Autodesk Inventor part; units mm, degrees
ref_plane "YZ Plane" through (0, 0, 0) normal (1, 0, 0) x (0, 1, 0)
ref_plane "XZ Plane" through (0, 0, 0) normal (0, 1, 0) x (-1, 0, 0)
ref_plane "XY Plane" through (0, 0, 0) normal (0, 0, 1) x (1, 0, 0)
sketch "スケッチ1" plane through (0, 0, 0) normal (0, 0, 1) x (1, 0, 0)
  circle A0 centre (0, 0) radius 3.1
  circle A1 centre (0, 0) radius 2.5
  circle A2 centre (0, 0) radius 1
  dimension "d0" = 6.2
  dimension "d1" = 5
  dimension "d2" = 2
extrude "押し出し1" add sketch "スケッチ1" against normal blind 0.6 contours A0 | A1
extrude "押し出し2" add sketch "スケッチ1" along normal blind 1.9 contours A1
sketch "スケッチ2" plane through (0, 0, -0.6) normal (0, 0, -1) x (-1, 0, 0)
  circle A0 centre (0, 0) radius 2.75
  circle A1 centre (0, 0) radius 1.5
  circle A2 centre (0, 0) radius 2.625
  circle A3 centre (0, 0) radius 1.625
  dimension "d7" = 5.5
  dimension "d8" = 3
  dimension "d11" = 5.25
  dimension "d12" = 3.25
extrude "押し出し4" cut sketch "スケッチ2" against normal blind 0.5 contours A3
extrude "押し出し5" cut sketch "スケッチ2" against normal blind 0.5 contours A0
properties part number "ベアリング"
Read the model definition and answer for the solid it produces. Units are mm, in the model's axes. A direction names the side the tool comes from. Give positions to 0.01 mm unless a question says otherwise; leave off trailing zeros. Loops run counter-clockwise (first coordinate to the right, second up) from the corner with the lowest first, then second, coordinate; pieces in that order, holes last.
Item 1: The part is cut by section D-D (y = 1.75). Write down the section's boundary in (x, z), and give its area (3 significant figures).
Item 2: For faces 4 (the cylindrical face through (-0.54, 2.44, 0.94)), 5 (the flat face through (1, -1, 1.9)), determine the directions among +Z, -Z, +X, -X, +Y, -Y from which every point of the face is accessible in a straight line to the end or side of a thin tool.
Item 3: The part is cut by section A-A (x = 0). Write down the section's boundary in (y, z) (3 decimals).
Item 4: The part is cut by section C-C (z = 0.6). Write down the section's boundary in (x, y).
Item 5: Each of these flat-tipped pins is pushed along its axis until it touches: pin 1 Ø1 at (y, z) = (-1, 0) entering from +X; pin 2 Ø1.5 at (x, z) = (-1, 1) entering from +Y. Where does it stop, or does it pass through?
Item 6: The mould has two halves that part along Y. Classify faces 1 (the flat face through (0, -2, -0.6)), 2 (the cylindrical face through (1.43, -2.75, -0.3)), 3 (the cylindrical face through (0, 1, 1)): released by +Y, released by -Y, zero draft, split by the parting line, or undercut.
Item 7: Find the intervals of material crossed by line 1 along Y through (x, z) = (0, 0.55); line 2 along X through (y, z) = (-2, 1), in increasing order.
Taken from the geometry:
1. outline: (-2.56, -0.6) - (-2.12, -0.6) - (-2.12, -0.1) - (-1.96, -0.1) - (-1.96, -0.6) - (1.96, -0.6) - (1.96, -0.1) - (2.12, -0.1) - (2.12, -0.6) - (2.56, -0.6) - (2.56, 0) - (1.79, 0) - (1.79, 1.9) - (-1.79, 1.9) - (-1.79, 0) - (-2.56, 0) - close
1. area: 9.69 mm2
2. face 4: +Z
2. face 5: +Z, +X, -X, +Y, -Y
3. outline: (-3.1, -0.6) - (-2.75, -0.6) - (-2.75, -0.1) - (-2.625, -0.1) - (-2.625, -0.6) - (-1.625, -0.6) - (-1.625, -0.1) - (-1.5, -0.1) - (-1.5, -0.6) - (-1, -0.6) - (-1, 1.9) - (-2.5, 1.9) - (-2.5, 0) - (-3.1, 0) - close; (1, -0.6) - (1.5, -0.6) - (1.5, -0.1) - (1.625, -0.1) - (1.625, -0.6) - (2.625, -0.6) - (2.625, -0.1) - (2.75, -0.1) - (2.75, -0.6) - (3.1, -0.6) - (3.1, 0) - (2.5, 0) - (2.5, 1.9) - (1, 1.9) - close
4. outline: circle Ø5 at (0, 0); hole circle Ø2 at (0, 0)
5. pin 1: stops at x = 3.06
5. pin 2: stops at y = 2.49
6. face 1: zero draft
6. face 2: split by the parting line
6. face 3: undercut
7. line 1: y = -2.5 to -1, 1 to 2.5
7. line 2: x = -1.5 to 1.5
